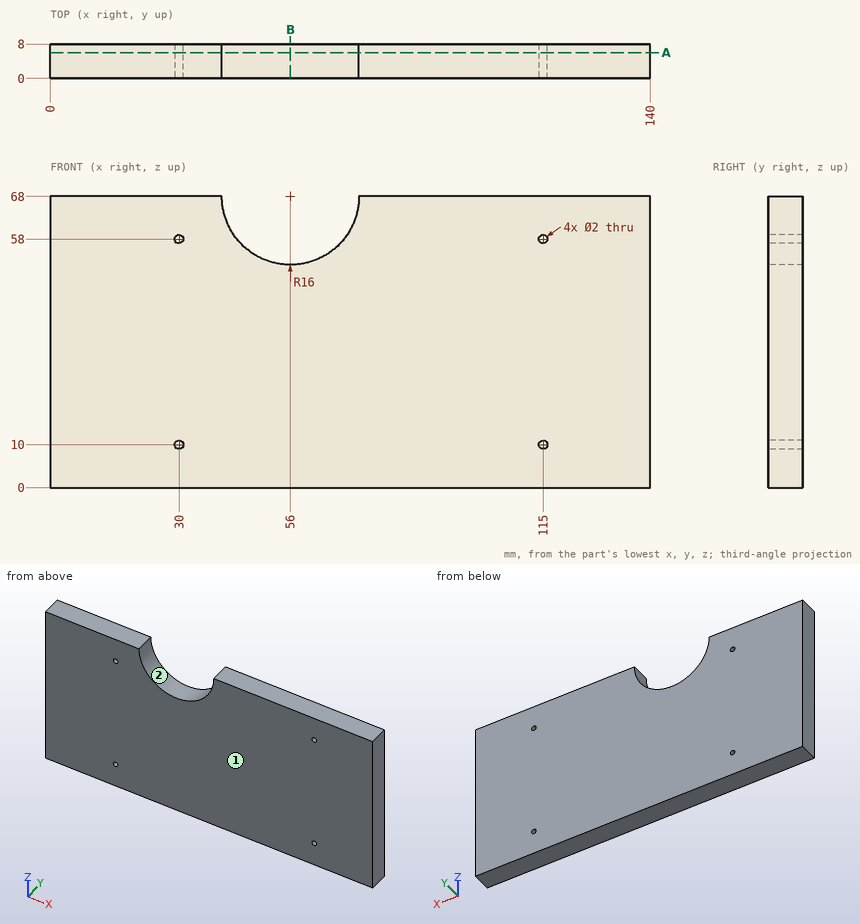
The drawing under review shows one solid part. Ordinate dimensions are in mm from its lowest x, y, z. Give positions to 0.01 mm unless a question says otherwise; leave off trailing zeros. Order: outer loops, then holes, each group sorted by start corner. A loop starts at its lowest first (then second) coordinate and runs counter-clockwise, first axis right, second up. Notation, with made-up numbers: M -37,-40 L 7,-40 A22 cw 7,-10 Z; hole C 34.5,28 d6. An arc over 180 degrees is marked long. One line per question, with ' | ' between items. Start each with the question number.
Q1. For L1, parallel to Z at x = 115, y = 5; L2, parallel to X at y = 6, z = 10; L3, parallel to X at y = 2.5, z = 58.5, list the stretches that pass through material, from the lowest coordinate up. Write a range as [from, to].
Q2. The part is to be moulded in two halves that separate along X. For the marked faces 1 and 2, say which applies: +X half, -X half, draft (parallel to the pull), parting line (faces both ways), or undercut.
Q3. We need section B-B (x = 56). Write out the cut boundary in (y, z), plus the area to 3 significant figures.
Q4. We need section A-A (y = 6). Write out the cut boundary in (x, z), plus the area to 3 significant figures.
Q5. For pin 1 Ø1.6 at (x, z) = (30, 58) entering from +Y, flat-tipped, find the tip position at first contact; note if it passes through.
Returned:
1) L1: [0, 9], [11, 57], [59, 68] | L2: [0, 29], [31, 114], [116, 140] | L3: [0, 29.13], [30.87, 43.13], [68.87, 114.13], [115.87, 140]
2) face 1: draft | face 2: undercut
3) outline: M 0,0 L 8,0 L 8,52 L 0,52 Z | area: 416 mm2
4) outline: M 0,0 L 140,0 L 140,68 L 72,68 A16 cw 40,68 L 0,68 Z; hole C 30,10 d2; hole C 30,58 d2; hole C 115,10 d2; hole C 115,58 d2 | area: 9,110 mm2
5) pin 1: through
